```python
from build123d import *

# Parameters (mm, degrees)
F0_W     = 304.8
F0_H     = 228.6
F1_DEPTH = 19.05
F3_DEPTH = 9.525
F4_W     = 193.675
F4_H     = 19.05
F5_DEPTH = 9.525
F6_W     = 193.675
F6_H     = 19.05
F7_DEPTH = 9.525


with BuildPart() as f1:
    # F0 (on Top) → F1 (new body)
    with BuildSketch(Plane.XY):
        Rectangle(F0_W, F0_H)
    extrude(amount=F1_DEPTH)

    # F2 (on face) → F3 (cut)
    with BuildSketch(Plane.XY.offset(19.05)):
        Polygon((188.140169, -88.9), (188.140169, -79.375), (-188.140169, -79.375), (-188.140169, -88.9), (0, -88.9), align=None)
    extrude(amount=-F3_DEPTH, mode=Mode.SUBTRACT)

    # F4 (on face) → F5 (cut)
    with BuildSketch(Plane(origin=(-152.4, 0, 0), x_dir=(0, -1, 0), z_dir=(-1, 0, 0))):
        with Locations((-17.4625, 19.05)):
            Rectangle(F4_W, F4_H)
    extrude(amount=-F5_DEPTH, mode=Mode.SUBTRACT)

    # F6 (on face) → F7 (cut)
    with BuildSketch(Plane.YZ.offset(152.4)):
        with Locations((17.4625, 19.05)):
            Rectangle(F6_W, F6_H)
    extrude(amount=-F7_DEPTH, mode=Mode.SUBTRACT)


solid = f1.part
```
The listing builds one solid part. Answer for the finished solid, in the listing's coordinates (mm). A direction names the side the tool comes from. Give positions to 0.01 mm unless a question says otherwise; leave off trailing zeros. Loops run counter-clockwise (first coordinate to the right, second up) from the corner with the lowest first, then second, coordinate; pieces in that order, holes last. Notation, with made-up numbers: (-24, 3) - (-4, 3) arc R9 ccw to (-4, 8) - close; hole circle Ø8 at (62.25, 81). An arc over 180 degrees is marked (long way). Return JSON: item names as keys, results as strings. Group by question number.
1. Find section B-B (x = -123). Write down the section's boundary in (y, z) (3 decimals).
2. Given pin 1 Ø3 at (y, z) = (-26, 16) entering from +X (3 decimals); pin 2 Ø4 at (y, z) = (19, 14) entering from -X (3 decimals), each flat-ended and moving along its own axis, determine where each tip first touches the part or whether it passes through.
3. Straight lines are drawn through the part: line 1 (Y direction, x = 121, z = 10.25) (3 decimals); line 2 (X direction, y = 98, z = 15) (3 decimals). For each, find the intervals that lie inside material, in ascending order. Write a range as [from, to].
4. Determine the mould class of faces 1 (the flat face through (-2, 2, 0)), 2 (the flat face through (-2, 114.3, 9)), 3 (the flat face through (2, -79.375, 14)) for opening direction Y: pulls with the +Y half, pulls with the -Y half, needs draft (parallel to the pull), parting line crosses it, or undercut.
5. Find section A-A (z = 12.75). Write down the section's boundary in (x, y) (3 decimals), then the cut area to 3 significant figures.
6. Which of the six approach directions +Z, -Z, +X, -X, +Y, -Y give full straight-line access (tool end or side, diameter ignored) to faces 4 (the flat face through (-2, -88.9, 14)), 5 (the flat face through (-152.4, -2, 5)), 6 (the flat face through (142.875, 16, 14)), 7 (the flat face through (-2, -114.3, 9)), 8 (the flat face through (-142.875, 19, 14))?
7. Find section C-C (y = -33). Write down the section's boundary in (x, z) (3 decimals).
Verdict:
{
 "1": {"outline": "(-114.3, 0) - (114.3, 0) - (114.3, 19.05) - (-79.375, 19.05) - (-79.375, 9.525) - (-88.9, 9.525) - (-88.9, 19.05) - (-114.3, 19.05) - close"},
 "2": {"pin 1": "stops at x = 142.875", "pin 2": "stops at x = -142.875"},
 "3": {"line 1": "y = [-114.3, -88.9], [-79.375, 114.3]", "line 2": "x = [-142.875, 142.875]"},
 "4": {"face 1": "needs draft", "face 2": "pulls with the +Y half", "face 3": "undercut"},
 "5": {"outline": "(-152.4, -114.3) - (152.4, -114.3) - (152.4, -88.9) - (-152.4, -88.9) - close; (-142.875, -79.375) - (142.875, -79.375) - (142.875, 114.3) - (-142.875, 114.3) - close", "area": "63,100 mm^2"},
 "6": {"face 4": "+Z, +X, -X", "face 5": "+Z, -Z, -X, +Y, -Y", "face 6": "+Z, +X, +Y", "face 7": "+Z, -Z, +X, -X, -Y", "face 8": "+Z, -X, +Y"},
 "7": {"outline": "(-152.4, 0) - (152.4, 0) - (152.4, 9.525) - (142.875, 9.525) - (142.875, 19.05) - (-142.875, 19.05) - (-142.875, 9.525) - (-152.4, 9.525) - close"}
}
